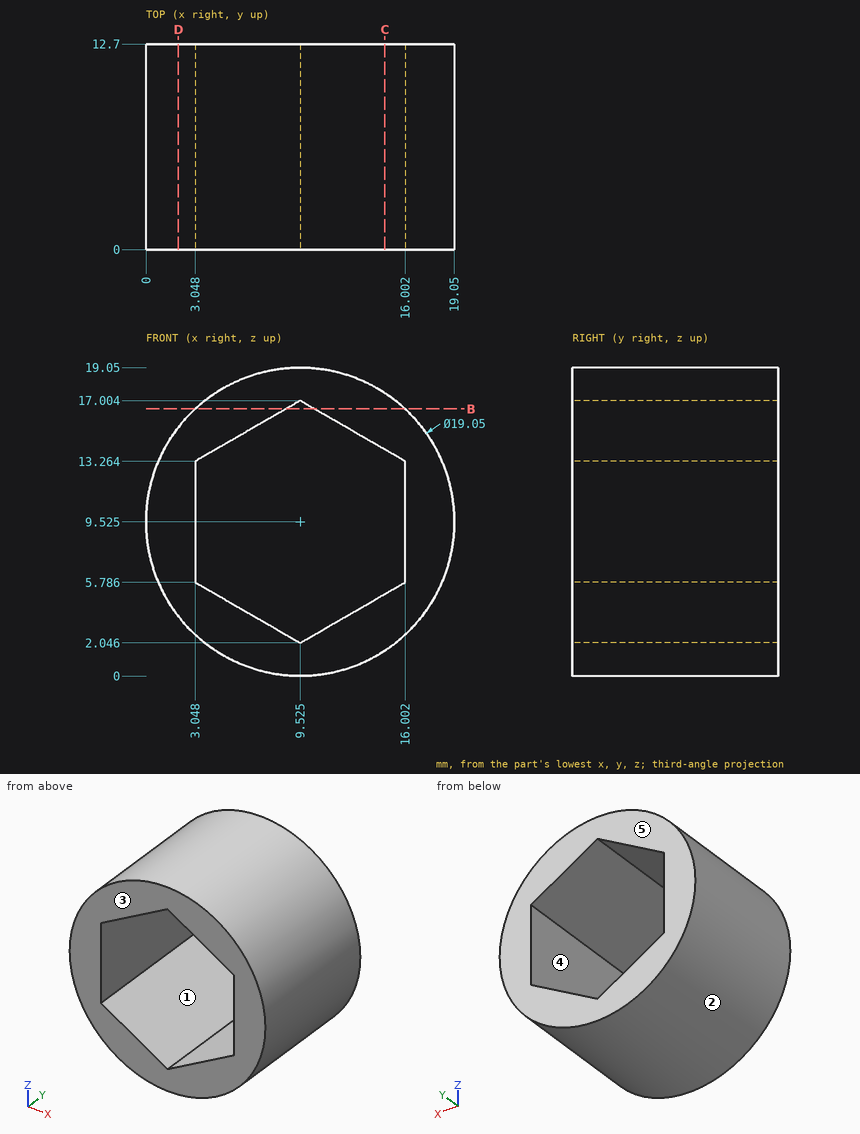
Verification items for this drawing (mm, ordinates from the low corner). A direction names the side the tool comes from. Give positions to 0.01 mm unless a question says otherwise; leave off trailing zeros. Loops run counter-clockwise (first coordinate to the right, second up) from the corner with the lowest first, then second, coordinate; pieces in that order, holes last.
1. Cross-section at D-D on x = 2. Record the cut outline in (y, z) (1 decimal).
Derived:
outline: (0, 3.7) - (12.7, 3.7) - (12.7, 15.4) - (0, 15.4) - close
2. Cross-section at C-C on x = 14.75. Record the cut outline in (y, z).
Derived:
outline: (0, 1.56) - (12.7, 1.56) - (12.7, 5.06) - (0, 5.06) - close; (0, 13.99) - (12.7, 13.99) - (12.7, 17.49) - (0, 17.49) - close
3. Material ranges on probe 1 along Z at (x, y) = (11.75, 2.25) (1 decimal); probe 2 along Z at (x, y) = (7.5, 9.75) (1 decimal); probe 3 along X at (y, z) = (3.5, 5.5) (1 decimal), recorded low to high.
Derived:
probe 1: z = 0.3 to 3.3, 15.7 to 18.8
probe 2: z = 0.2 to 3.2, 15.8 to 18.8
probe 3: x = 0.9 to 3.5, 15.5 to 18.2
4. Go/stop test with flat-tipped pins: P1, Ø3, axis at y = 3, z = 3, coming from the +X side; P2, Ø1, axis at x = 4, y = 1.5, coming from the -Z side; P3, Ø2, axis at x = 3, y = 10, coming from the +Z side (1 decimal). Record where each tip stops, or that it passes through.
Derived:
P1: stops at x = 17.62
P2: stops at z = 1.43
P3: stops at z = 17.3
5. Tool access check on the marked faces 4 and 5. Record the directions out of +Z, -Z, +X, -X, +Y, -Y that give a thin tool (end or side, any length) a straight path to the whole face; none if there is none.
Derived:
face 4: +Y, -Y
face 5: +Z, -Z, +X, -X, +Y
6. Cross-section at B-B on z = 16.5. Record the cut outline in (x, y).
Derived:
outline: (3.04, 0) - (8.65, 0) - (8.65, 12.7) - (3.04, 12.7) - close; (10.4, 0) - (16.01, 0) - (16.01, 12.7) - (10.4, 12.7) - close
7. Release check for a two-part mould opening along Z. For the marked faces 1, 2 and 3 record: +Z half, -Z half, draft (parallel to the pull), parting line (faces both ways), or undercut.
Derived:
face 1: undercut
face 2: parting line
face 3: draft
